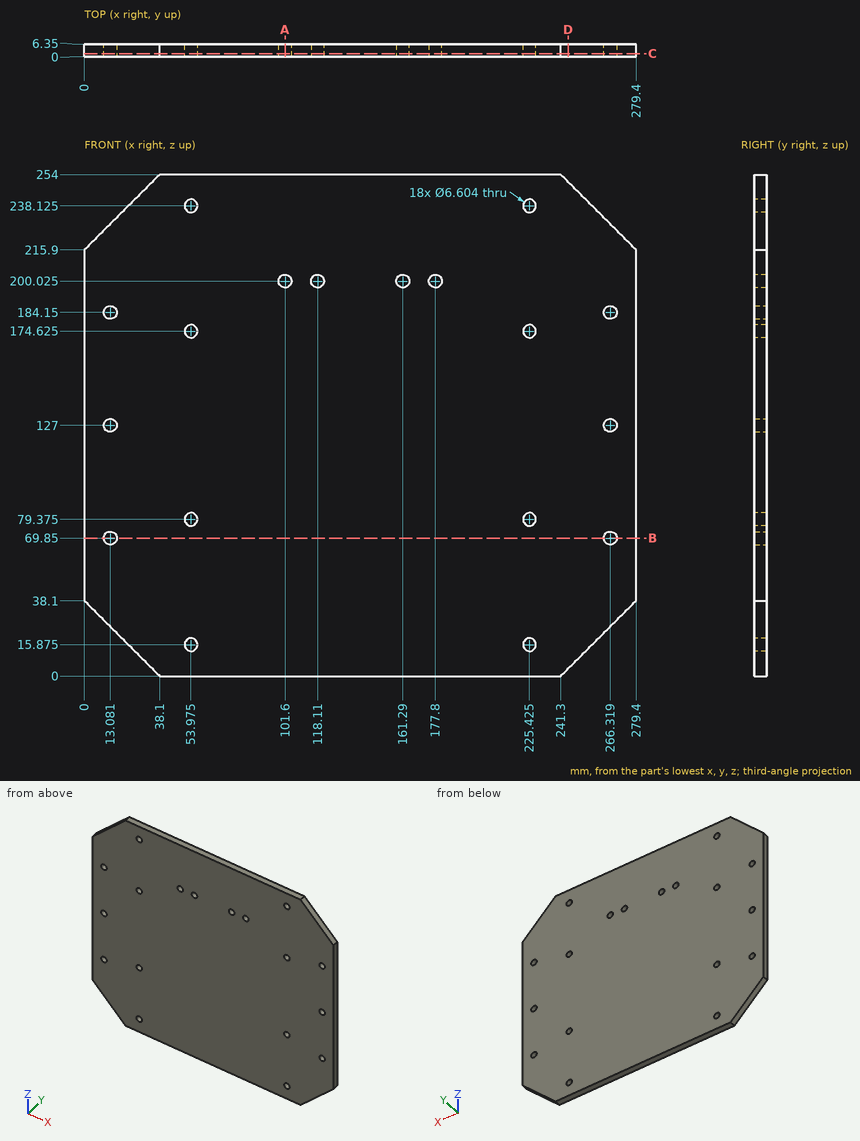
Geometry: see drawing. Coordinates: mm, zero at the bounding-box minimum. Coordinates: 2 decimals unless noted, no trailing zeros. Write each loop counter-clockwise with the first axis right and the second up, starting at its lowest first coordinate (ties: lowest second). Pieces come first, ordered by that corner, then holes. Notation, with made-up numbers: M -21.5,80 L 10.5,80 A23 cw 10.5,103 Z; hole C 0.5,27 d11. An arc over 180 degrees is marked long. Use CSV: the item, a comma, the result in double quotes. Start each with the question number.
1. Cut plane B-B on z = 69.85. Return the cut outline in (x, y).
2. First-contact query: P1, Ø5.5, axis at x = 13.081, z = 127, coming from the -Y side. Flat tip, straight axial feed; report the tip coordinate or a pass-through.
3. Ray query, probe 1 along X at (y, z) = (2.5, 184.15); probe 2 along X at (y, z) = (4, 202.5); probe 3 along Z at (x, y) = (264.5, 2.25). Return the intervals inside material, ascending.
4. Cut plane A-A on x = 101.6. Return the cut outline in (y, z).
5. Cut plane D-D on x = 245. Return the cut outline in (y, z), plus the area to 3 significant figures.
6. Cut plane C-C on y = 1.5. Count the separate pieces of the cut face and the enclosed holes in it, plus the area to 3 significant figures.
Entries:
1,outline,"M 0,0 L 9.78,0 L 9.78,6.35 L 0,6.35 Z; M 16.38,0 L 263.02,0 L 263.02,6.35 L 16.38,6.35 Z; M 269.62,0 L 279.4,0 L 279.4,6.35 L 269.62,6.35 Z"
2,P1,"through"
3,probe 1,"0 to 9.78, 16.38 to 263.02, 269.62 to 279.4"
3,probe 2,"0 to 99.41, 103.79 to 115.92, 120.3 to 159.1, 163.48 to 175.61, 179.99 to 279.4"
3,probe 3,"23.2 to 67.09, 72.61 to 124.24, 129.76 to 181.39, 186.91 to 230.8"
4,outline,"M 0,0 L 6.35,0 L 6.35,196.72 L 0,196.72 Z; M 0,203.33 L 6.35,203.33 L 6.35,254 L 0,254 Z"
5,outline,"M 0,3.7 L 6.35,3.7 L 6.35,250.3 L 0,250.3 Z"
5,area,"1,570 mm²"
6,separate pieces,"1"
6,enclosed holes,"18"
6,area,"67,400 mm²"
